Here's the drawing with two shaded views (mm, measured from the low corner). I have some questions. A direction names the side the tool comes from. Give positions to 0.01 mm unless a question says otherwise; leave off trailing zeros. Loops run counter-clockwise (first coordinate to the right, second up) from the corner with the lowest first, then second, coordinate; pieces in that order, holes last. Notation, with made-up numbers: (-9, -30.75) -> (28, -30.75) arc R15 ccw to (28, -12.75) -> close; hole circle Ø5 at (0.5, 32). An arc over 180 degrees is marked (long way). Answer in a Markdown table with one row per item. Add a question column.
Item 1: Which directions (+Z, -Z, +X, -X, +Y, -Y) give clear straight access to the entire face, cutting with the end or side of a thin tool? Please do the marked faces 1, 2 and 3.
Item 2: If we section it at D-D (y = 27): Write out the boundary of the cut face in (x, z).
Item 3: If we section it at A-A (y = 10): Write out the boundary of the cut face in (x, z).
Item 4: If we section it at B-B (x = 3.05): Write out the boundary of the cut face in (y, z), then the cut area to 3 significant figures.
Item 5: If I drill on line 1 (Y direction, x = 2.3, z = 0.25); line 2 (X direction, y = 19, z = 0.85); line 3 (X direction, y = 27.5, z = 2.4), over which ranges is the centre line in solid material (lowest first)?
Item 6: If we section it at C-C (z = 3.15): Write out the boundary of the cut face in (x, y) (1 decimal), then the cut area to 3 significant figures.
Item 7: For P1, Ø1.5, axis at x = 1.5, z = 2.5, coming from the -Y side, with a flat end and sliding along its axis, tell me the tip position at first contact or that it passes through.
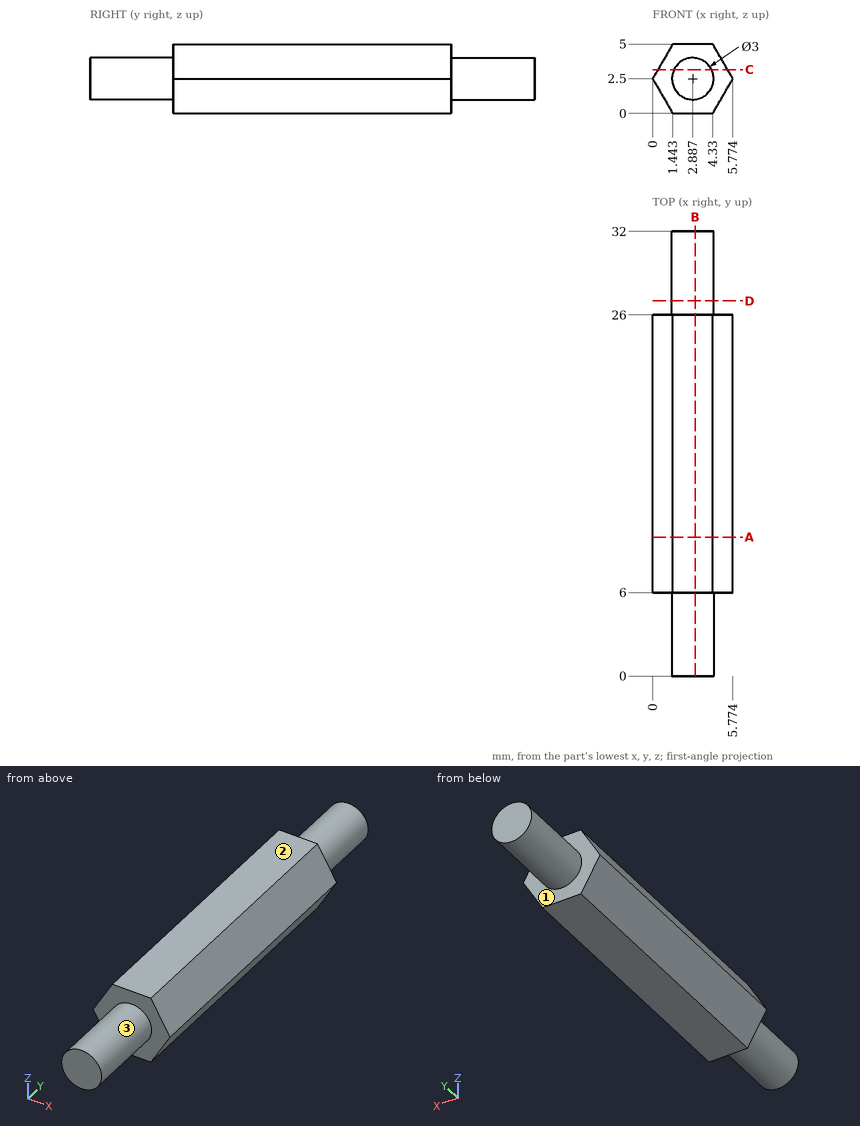
Recorded:
| question | item | result |
|---|---|---|
| 1 | face 1 | +Y |
| 1 | face 2 | +Z, +X, -X, +Y, -Y |
| 1 | face 3 | -Y |
| 2 | outline | circle Ø3 at (2.89, 2.5) |
| 3 | outline | (0, 2.5) -> (1.44, 0) -> (4.33, 0) -> (5.77, 2.5) -> (4.33, 5) -> (1.44, 5) -> close |
| 4 | outline | (0, 1.01) -> (6, 1.01) -> (6, 0) -> (26, 0) -> (26, 1.01) -> (32, 1.01) -> (32, 3.99) -> (26, 3.99) -> (26, 5) -> (6, 5) -> (6, 3.99) -> (0, 3.99) -> close |
| 4 | area | 136 mm^2 |
| 5 | line 1 | y = 6 to 26 |
| 5 | line 2 | x = 0.95 to 4.82 |
| 5 | line 3 | x = 1.39 to 4.38 |
| 6 | outline | (0.4, 6) -> (1.5, 6) -> (1.5, 0) -> (4.2, 0) -> (4.2, 6) -> (5.4, 6) -> (5.4, 26) -> (4.2, 26) -> (4.2, 32) -> (1.5, 32) -> (1.5, 26) -> (0.4, 26) -> close |
| 6 | area | 133 mm^2 |
| 7 | P1 | stops at y = 0 |
